from build123d import *

# Parameters (mm, degrees)
SKETCH1_W              = 25.4
SKETCH1_H              = 25.4
SKETCH1_W_2            = 20.32
SKETCH1_H_2            = 20.32
BOSS_EXTRUDE1_DEPTH    = 101.6
SKETCH4_R              = 3.175
CUT_EXTRUDE3_DEPTH     = 25.4
SKETCH5_R              = 3.175
CUT_EXTRUDE4_DEPTH     = 25.4
SKETCH6_R              = 1.27
CUT_EXTRUDE6_DEPTH     = 25.4
F_10_CLEARANCE_HOLE1_D = 5.1054


with BuildPart() as part:
    # Sketch1 → Boss-Extrude1 (new, symmetric)
    with BuildSketch(Plane(origin=(0, 0, 0), x_dir=(1, 0, 0), z_dir=(0, 1, 0))):
        Rectangle(SKETCH1_W, SKETCH1_H)
        Rectangle(SKETCH1_W_2, SKETCH1_H_2, mode=Mode.SUBTRACT)
    extrude(amount=BOSS_EXTRUDE1_DEPTH, both=True)

    # Sketch4 → Cut-Extrude3 (cut)
    with BuildSketch(Plane.XY.offset(12.7)):
        with Locations((0, 63.5)):
            Circle(SKETCH4_R)
        with Locations((0, -63.5)):
            Circle(SKETCH4_R)
    extrude(amount=-CUT_EXTRUDE3_DEPTH, mode=Mode.SUBTRACT)

    # Sketch5 → Cut-Extrude4 (cut)
    with BuildSketch(Plane.XY.offset(12.7)):
        with Locations((0, 25.4)):
            Circle(SKETCH5_R)
        with Locations((0, -25.4)):
            Circle(SKETCH5_R)
    extrude(amount=-CUT_EXTRUDE4_DEPTH, mode=Mode.SUBTRACT)

    # Sketch6 → Cut-Extrude6 (cut)
    with BuildSketch(Plane.XY.offset(12.7)):
        with Locations((0, -88.9)):
            Circle(SKETCH6_R)
        with Locations((0, -52.959)):
            Circle(SKETCH6_R)
    extrude(amount=-CUT_EXTRUDE6_DEPTH, mode=Mode.SUBTRACT)

    # #10 Clearance Hole1 (through all)
    with Locations(Plane(origin=(0, 0, -12.7), x_dir=(-1, 0, 0), z_dir=(0, 0, -1))):
        with Locations((0, -52.959), (0, -88.9)):
            Hole(F_10_CLEARANCE_HOLE1_D / 2)


solid = part.part
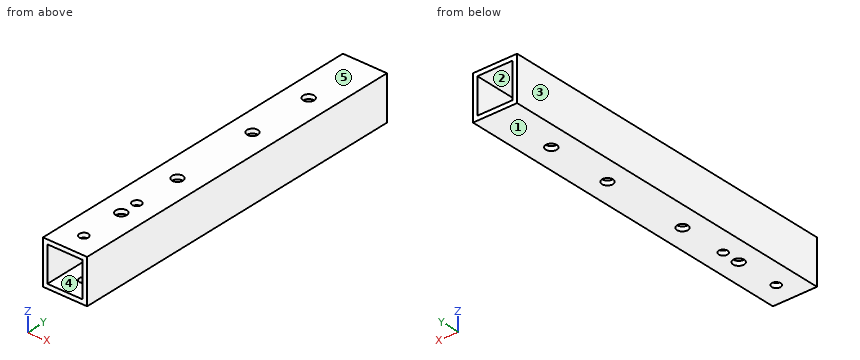
Build history of the part. All positions in model axes, mm. Face numbers are marked on the shaded views. A direction names the side the tool comes from. Give positions to 0.01 mm unless a question says otherwise; leave off trailing zeros. Loops run counter-clockwise (first coordinate to the right, second up) from the corner with the lowest first, then second, coordinate; pieces in that order, holes last. Notation, with made-up numbers: (15, 38.5) -> (20, 38.5) arc R19 ccw to (20, 62.5) -> close; hole circle Ø4 at (-39.5, 51.25). An arc over 180 degrees is marked (long way). Answer in a Markdown table with one row per item.
Item 1: Tool access for the marked faces 1 and 2: list every direction of +Z, -Z, +X, -X, +Y, -Y with a clear straight run to the whole face (end or side of a thin tool).
Findings below:
| item | result |
|---|---|
| face 1 | -Z, +X, -X, +Y, -Y |
| face 2 | +Y, -Y |
Item 2: Slice it at A-A on y = -25.4. Write the cut outline in (x, z) (3 decimals), plus the area to 3 significant figures.
Findings below:
| item | result |
|---|---|
| outline | (-12.7, -12.7) -> (-3.175, -12.7) -> (-3.175, -10.16) -> (-10.16, -10.16) -> (-10.16, 10.16) -> (-3.175, 10.16) -> (-3.175, 12.7) -> (-12.7, 12.7) -> close; (3.175, -12.7) -> (12.7, -12.7) -> (12.7, 12.7) -> (3.175, 12.7) -> (3.175, 10.16) -> (10.16, 10.16) -> (10.16, -10.16) -> (3.175, -10.16) -> close |
| area | 200 mm² |
Item 3: Probe line 1 along X through (y, z) = (-73, 7); line 2 along X through (y, z) = (27.5, 10.75). List the from-to ranges inside material, lowest first. Write a range as [from, to].
Findings below:
| item | result |
|---|---|
| line 1 | x = [-12.7, -10.16], [10.16, 12.7] |
| line 2 | x = [-12.7, -2.38], [2.38, 12.7] |
Item 4: Slice it at C-C on z = -0.25. Write the cut outline in (x, y).
Findings below:
| item | result |
|---|---|
| outline | (-12.7, -101.6) -> (-10.16, -101.6) -> (-10.16, 101.6) -> (-12.7, 101.6) -> close; (10.16, -101.6) -> (12.7, -101.6) -> (12.7, 101.6) -> (10.16, 101.6) -> close |
Item 5: Mould opens along X. For the marked faces 3, 4 and 5 say: pulls with the +X half, pulls with the -X half, needs draft (parallel to the pull), parting line crosses it, or undercut.
Findings below:
| item | result |
|---|---|
| face 3 | pulls with the -X half |
| face 4 | undercut |
| face 5 | needs draft |
Item 6: Slice it at B-B on x = 7.25. Write the cut outline in (y, z).
Findings below:
| item | result |
|---|---|
| outline | (-101.6, -12.7) -> (101.6, -12.7) -> (101.6, -10.16) -> (-101.6, -10.16) -> close; (-101.6, 10.16) -> (101.6, 10.16) -> (101.6, 12.7) -> (-101.6, 12.7) -> close |
